Answer from the drawing. Dimensions are ordinates in mm from the lowest x, y and z of the part. A direction names the side the tool comes from. Round coordinates to 2 decimals unless told otherwise and drop trailing zeros. Loops run counter-clockwise (first coordinate to the right, second up) from the corner with the lowest first, then second, coordinate; pieces in that order, holes last. Notation, with made-up numbers: (27.5, 46.25) - (40.5, 46.25) arc R16 cw to (40.5, 59.25) - close; hole circle Ø8 at (81.25, -11.75). An arc over 180 degrees is marked (long way). Write item = value, one per line. Start each with the question number.
1) Section A-A, the plane z = 11 is taken. Determine the outline of the cut face in (x, y).
2) Section B-B, the plane x = 50 is taken. Determine the outline of the cut face in (y, z), and give its area (3 significant figures).
3) For a pull along Y with two mould halves and no side action, classify the marked faces 3, 4, 5 and 6 as released by +Y, released by -Y, zero draft, split by the parting line, or undercut.
4) A tool of negligible diameter and unlimited length cuts with its end or side. For the marked faces 1 and 2, from which of +Z, -Z, +X, -X, +Y, -Y can it reach the whole face along a straight path? Write none if from no direction.
5) Section C-C, the plane y = 17.5 is taken. Determine the outline of the cut face in (x, z).
6) Straight lines are drawn through the part: line 1 along Y through (x, z) = (85, 10.75); line 2 along X through (y, z) = (49.5, 3.25); line 3 along Z through (x, y) = (76, 23). For each, find the intervals that lie inside material, in ascending order.
7) Given pin 1 Ø12 at (x, y) = (38.5, 19.5) entering from +Z, flat-ended and moving along its own axis, determine where the tip first touches the part or whether it passes through.
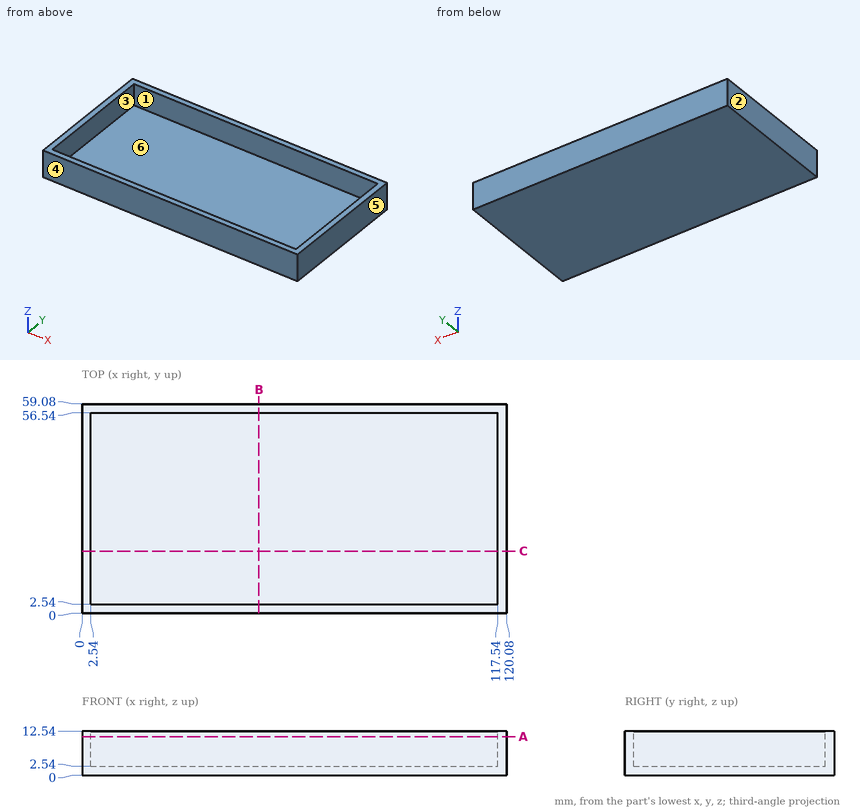
Geometry check:
q1.outline = (0, 0) - (120.08, 0) - (120.08, 59.08) - (0, 59.08) - close; hole (2.54, 2.54) - (117.54, 2.54) - (117.54, 56.54) - (2.54, 56.54) - close
q2.outline = (0, 0) - (59.08, 0) - (59.08, 12.54) - (56.54, 12.54) - (56.54, 2.54) - (2.54, 2.54) - (2.54, 12.54) - (0, 12.54) - close
q2.area = 201 mm2
q3.face_3 = undercut
q3.face_4 = released by -Y
q3.face_5 = zero draft
q3.face_6 = undercut
q4.face_1 = +Z
q4.face_2 = +Z, -Z, -X, +Y, -Y
q5.outline = (0, 0) - (120.08, 0) - (120.08, 12.54) - (117.54, 12.54) - (117.54, 2.54) - (2.54, 2.54) - (2.54, 12.54) - (0, 12.54) - close
q6.line_1 = 0 to 2.54, 56.54 to 59.08
q6.line_2 = 0 to 2.54, 117.54 to 120.08
q6.line_3 = 0 to 2.54
q7.pin_1 = 2.54
